Design review of the part built by this model. Coordinates are the model's own, in mm. Face numbers are marked on the shaded views. A direction names the side the tool comes from. Give positions to 0.01 mm unless a question says otherwise; leave off trailing zeros. Order: outer loops, then holes, each group sorted by start corner. A loop starts at its lowest first (then second) coordinate and runs counter-clockwise, first axis right, second up. Notation, with made-up numbers: M 77.5,22.5 L 84.5,22.5 A32 ccw 84.5,57.5 Z; hole C 73.25,76.5 d7. An arc over 180 degrees is marked long. Answer as a JSON object with one key per item and string values.
from build123d import *

# Parameters (mm, degrees)
EXTRUDE_THIN1_DEPTH     = 564
CUT_EXTRUDE2_DEPTH      = 594.060705156
CUT_EXTRUDE2_DEPTH_BACK = 594.060705156
SKETCH3_W               = 165
SKETCH3_H               = 220
FILLET1_R               = 20


with BuildPart() as part:
    # Sketch1 → Extrude-Thin1 (new body)
    with BuildSketch(Plane(origin=(0, 0, 0), x_dir=(1, 0, 0), z_dir=(0, 1, 0))):
        with BuildLine():
            Line((-159, -80), (-159, -20))
            ThreePointArc((-159, -20), (-153.142135624, -5.857864376), (-139, 0))
            Line((-139, 0), (139, 0))
            ThreePointArc((139, 0), (153.142135624, -5.857864376), (159, -20))
            Line((159, -20), (159, -80))
            Line((159, -80), (163, -80))
            Line((163, -80), (163, -20))
            ThreePointArc((163, -20), (155.970562748, -3.029437252), (139, 4))
            Line((139, 4), (-139, 4))
            ThreePointArc((-139, 4), (-155.970562748, -3.029437252), (-163, -20))
            Line((-163, -20), (-163, -80))
            Line((-163, -80), (-159, -80))
        make_face()
    extrude(amount=EXTRUDE_THIN1_DEPTH)

    # Sketch3 → Cut-Extrude2 (cut, two sides: drawn at the far end of the back side and taken through both)
    with BuildSketch(Plane(origin=(0, 0, -4), x_dir=(-1, 0, 0), z_dir=(0, 0, -1)).offset(-CUT_EXTRUDE2_DEPTH_BACK)):
        with Locations((0, 110)):
            Rectangle(SKETCH3_W, SKETCH3_H)
    extrude(amount=CUT_EXTRUDE2_DEPTH + CUT_EXTRUDE2_DEPTH_BACK, mode=Mode.SUBTRACT)

    # Fillet1
    fillet1_edges = [part.edges().sort_by_distance(p)[0] for p in [
        (-82.5, 0, -2),
        (82.5, 0, -2),
        (82.5, 220, -2),
        (-82.5, 220, -2),
    ]]
    fillet(fillet1_edges, radius=FILLET1_R)


solid = part.part
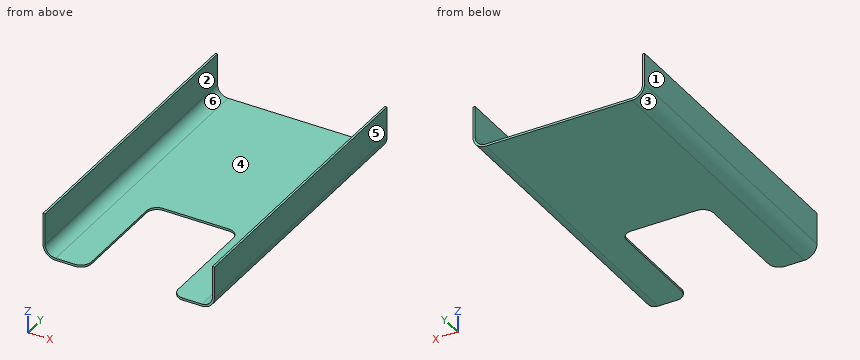
(1) We need section A-A (z = 58). Write out the cut boundary in (x, y).
Checked values:
{"outline": "M -163,0 L -159,0 L -159,564 L -163,564 Z; M 159,0 L 163,0 L 163,564 L 159,564 Z"}
(2) We need section C-C (y = 286). Write out the cut boundary in (x, z), plus the area to 3 significant figures.
Checked values:
{"outline": "M -163,20 A24 ccw -139,-4 L 139,-4 A24 ccw 163,20 L 163,80 L 159,80 L 159,20 A20 cw 139,0 L -139,0 A20 cw -159,20 L -159,80 L -163,80 Z", "area": "1,870 mm^2"}
(3) To check wall thickness, follow L1, parallel to X at y = 384, z = 20.5; L2, parallel to X at y = 415.5, z = 18; L3, parallel to Z at x = -17, y = 333.5. State the ranges of each line that lie inside material, in increasing order. Write a range as from..to.
Checked values:
{"L1": "x = -163..-159, 159..163", "L2": "x = -162.92..-158.9, 158.9..162.92", "L3": "z = -4..0"}
(4) We need section B-B (y = 96). Write out the cut boundary in (x, z).
Checked values:
{"outline": "M -163,20 A24 ccw -139,-4 L -82.5,-4 L -82.5,0 L -139,0 A20 cw -159,20 L -159,80 L -163,80 Z; M 82.5,-4 L 139,-4 A24 ccw 163,20 L 163,80 L 159,80 L 159,20 A20 cw 139,0 L 82.5,0 Z"}
(5) We need section D-D (x = 109.5). Write out the cut boundary in (y, z), plus the area to 3 significant figures.
Checked values:
{"outline": "M 0,-4 L 564,-4 L 564,0 L 0,0 Z", "area": "2,260 mm^2"}
(6) Tool access review of the marked faces 1 and 2: name each direction out of +Z, -Z, +X, -X, +Y, -Y from which nothing blocks a thin tool from reaching the whole face with its end or side.
Checked values:
{"face 1": "+Z, -Z, -X, +Y, -Y", "face 2": "+Z, +Y, -Y"}
(7) Insertion check: pin 1 (2 mm diameter, centred on y = 139, z = -2.5, fed in from +X); pin 2 (3 mm diameter, centred on x = 19, z = -2, fed in from -Y); pin 3 (12 mm diameter, centred on x = -7, y = 236, fed in from +Z). Each pin has a flat end and moves straight along its axis. Give the tip position at first contact, or say it passes through.
Checked values:
{"pin 1": "stops at x = 149.67", "pin 2": "stops at y = 220", "pin 3": "stops at z = 0"}
(8) Draft analysis for pull direction X (two halves, no side actions). For the marked faces 3, 4, 5 and 6, state which applies: +X half, -X half, draft (parallel to the pull), parting line (faces both ways), or undercut.
Checked values:
{"face 3": "-X half", "face 4": "undercut", "face 5": "+X half", "face 6": "undercut"}
